CAD build for the part. Positions are in the model's coordinates, mm. A direction names the side the tool comes from. Coordinates: 2 decimals unless noted, no trailing zeros. Write each loop counter-clockwise with the first axis right and the second up, starting at its lowest first coordinate (ties: lowest second). Pieces come first, ordered by that corner, then holes. Notation, with made-up numbers: (11.5, 43.5) - (67.5, 43.5) arc R5 cw to (67.5, 49.5) - close; hole circle Ø7 at (-9, 21.5). An arc over 180 degrees is marked (long way). Answer in a Markdown table with one row per item. Add a question column.
Q1. Band-saw the part on A-A (x = -18.25). List the corners of the cut face in (y, z).
Q2. Two-plate mould, pull along Z, no slides. Class faces 1 (the flat face through (-10, 2, -24.7)), 2 (the flat face through (-10, 2, -6.7)), 3 (the flat face through (-10, 1, -56)): +Z half, -Z half, draft (parallel to the pull), parting line (faces both ways), or undercut.
Q3. Band-saw the part on B-B (z = -31). List the corners of the cut face in (x, y), and give its area (3 significant figures).
Q4. 3-axis set-ups, long thin cutter, end or side, ignore diameter. For faces 4 (the flat face through (-10, 2, -42.7)), 5 (the flat face through (-1.25, -5, -52)), 6 (the flat face through (-8.1, 2, -8)): which of +Z, -Z, +X, -X, +Y, -Y reach the whole face in a straight line?
Q5. Drill centre lines: line 1 along Y through (x, z) = (-13.25, -52); line 2 along Y through (x, z) = (-15.75, -50.5); line 3 along Z through (x, y) = (-8, -3.5). Where is each one in solid material? Low to high. Write a range as from..to.
Q6. Band-saw the part on D-D (x = -10.25). List the corners of the cut face in (y, z), and give its area (3 significant figures).
Q7. Band-saw the part on C-C (y = -4.5). List the corners of the cut face in (x, z).
Q8. Pin check, flat tips, straight feed: pin 1 (0.7 mm diameter, centred on y = 2, z = -7.5, fed in from +X); pin 2 (0.7 mm diameter, centred on y = 2, z = -7.5, fed in from -X); pin 3 (4 mm diameter, centred on y = -8.5, z = -47, fed in from -X); pin 4 (10 mm diameter, centred on x = -7.5, z = -15.5, fed in from +Y). Stop position of each tip, or through.
Autodesk Inventor part; units mm, degrees
ref_plane "YZ Plane" through (0, 0, 0) normal (1, 0, 0) x (0, 1, 0)
ref_plane "XZ Plane" through (0, 0, 0) normal (0, 1, 0) x (-1, 0, 0)
ref_plane "XY Plane" through (0, 0, 0) normal (0, 0, 1) x (1, 0, 0)
sketch "Sketch2" plane through (0, 0, 0) normal (0, 1, 0) x (-1, 0, 0)
  line L0 (20, 0) -> (0, 0)
  line L1 (0, 0) -> (0, -56)
  line L2 (0, -56) -> (20, -56)
  line L3 (20, -56) -> (20, 0)
  line L4 (18.75, -50.75) -> (1.25, -50.75)
  line L5 (1.25, -50.75) -> (1.25, -53.25)
  line L6 (1.25, -53.25) -> (18.75, -53.25)
  line L7 (18.75, -53.25) -> (18.75, -50.75)
  line L8 (11.9, -6.7) -> (8.1, -6.7)
  line L9 (8.1, -6.7) -> (8.1, -9.3)
  line L10 (8.1, -9.3) -> (11.9, -9.3)
  line L11 (11.9, -9.3) -> (11.9, -6.7)
  line L12 (11.9, -42.7) -> (8.1, -42.7)
  line L13 (8.1, -42.7) -> (8.1, -45.3)
  line L14 (8.1, -45.3) -> (11.9, -45.3)
  line L15 (11.9, -45.3) -> (11.9, -42.7)
  line L16 (8.1, -27.3) -> (11.9, -27.3)
  line L17 (8.1, -24.7) -> (8.1, -27.3)
  line L18 (11.9, -24.7) -> (8.1, -24.7)
  line L19 (11.9, -27.3) -> (11.9, -24.7)
  line L20 (23.6892, -52) -> (-2.3247, -52) construction
  line L21 (10, -54.7987) -> (10, -48.1542) construction
  line L22 (10, 9.3713) -> (10, -46.1174) construction
  line L23 (11.7769, -8) -> (1.25, -8) construction
  line L24 (11.7769, -26) -> (1.25, -26) construction
  line L25 (11.7769, -44) -> (1.25, -44) construction
  dimension "d0" = 20
  dimension "d1" = 56
  dimension "d2" = 17.5
  dimension "d3" = 2.5
  dimension "d9" = 3.8
  dimension "d10" = 2.6
  dimension "d13" = 3.8
  dimension "d14" = 2.6
  dimension "d30" = 3.8
  dimension "d31" = 2.6
  dimension "d40" = 10
  dimension "d41" = 10
  dimension "d45" = 8.1
  dimension "d46" = 8
  dimension "d47" = 18
  dimension "d48" = 18
  dimension "d49" = 4
extrude "Extrusion1" add sketch "Sketch2" along normal blind 1.6 contours L3 L2 L1 L0 | L7 L6 L5 L4 | L11 L10 L9 L8 | L15 L14 L13 L12 | L17 L18 L19 L16
extrude "Extrusion3" add sketch "Sketch2" against normal blind 10 contours L7 L6 L5 L4
extrude "Extrusion4" add sketch "Sketch2" along normal blind 2.98 contours L11 L10 L9 L8 | L15 L14 L13 L12 | L17 L18 L19 L16
properties part number "Sensor_Board_dummy"
Checked values:
| question | item | result |
|---|---|---|
| 1 | outline | (-10, -53.25) - (0, -53.25) - (0, -56) - (1.6, -56) - (1.6, 0) - (0, 0) - (0, -50.75) - (-10, -50.75) - close |
| 2 | face 1 | undercut |
| 2 | face 2 | +Z half |
| 2 | face 3 | -Z half |
| 3 | outline | (-20, 0) - (0, 0) - (0, 1.6) - (-20, 1.6) - close |
| 3 | area | 32.0 mm² |
| 4 | face 4 | +X, -X, +Y |
| 4 | face 5 | +Z, -Z, +X, -Y |
| 4 | face 6 | +Z, -Z, +X, +Y |
| 5 | line 1 | y = -10..1.6 |
| 5 | line 2 | y = 0..1.6 |
| 5 | line 3 | z = -53.25..-50.75 |
| 6 | outline | (-10, -53.25) - (0, -53.25) - (0, -56) - (1.6, -56) - (1.6, -45.3) - (2.98, -45.3) - (2.98, -42.7) - (1.6, -42.7) - (1.6, -27.3) - (2.98, -27.3) - (2.98, -24.7) - (1.6, -24.7) - (1.6, -9.3) - (2.98, -9.3) - (2.98, -6.7) - (1.6, -6.7) - (1.6, 0) - (0, 0) - (0, -50.75) - (-10, -50.75) - close |
| 6 | area | 125 mm² |
| 7 | outline | (-18.75, -53.25) - (-1.25, -53.25) - (-1.25, -50.75) - (-18.75, -50.75) - close |
| 8 | pin 1 | stops at x = -8.1 |
| 8 | pin 2 | stops at x = -11.9 |
| 8 | pin 3 | passes through |
| 8 | pin 4 | stops at y = 1.6 |
